```python
from build123d import *

# Parameters (mm, degrees)
SKETCH1_W           = 50
SKETCH1_H           = 50
BOSS_EXTRUDE1_DEPTH = 85
SKETCH2_R           = 5
BOSS_EXTRUDE2_DEPTH = 30
FILLET1_R           = 5
FILLET2_R           = 5
SKETCH3_W           = 70
SKETCH3_H           = 70
BOSS_EXTRUDE3_DEPTH = 10
FILLET3_R           = 5
SKETCH4_R           = 2.5
CUT_EXTRUDE1_DEPTH  = 10


with BuildPart() as part:
    # Sketch1 → Boss-Extrude1 (new body)
    with BuildSketch(Plane(origin=(0, 0, 0), x_dir=(1, 0, 0), z_dir=(0, 1, 0))):
        Rectangle(SKETCH1_W, SKETCH1_H)
    extrude(amount=BOSS_EXTRUDE1_DEPTH)

    # Sketch2 → Boss-Extrude2 (add)
    with BuildSketch(Plane.XZ):
        with Locations(Location((0, 0, 0), (0, 0, 90))):
            Circle(SKETCH2_R)
    extrude(amount=BOSS_EXTRUDE2_DEPTH)

    # Fillet1
    fillet1_edges = [part.edges().sort_by_distance(p)[0] for p in [
        (0, 85, 25),
        (0, 0, 25),
        (25, 42.5, 25),
        (-25, 42.5, 25),
    ]]
    fillet(fillet1_edges, radius=FILLET1_R)

    # Fillet2
    # the kernel refuses this fillet: 5 mm, written as the material it takes off along each edge
    with BuildSketch(Plane(origin=(-20, 80, 20), x_dir=(0, 1, 0), z_dir=(-1, 0, 0))) as fillet2_piece_1_section:
        Polygon((0, 0), (FILLET2_R, 0), (FILLET2_R, -FILLET2_R), (0, -FILLET2_R), align=None)
    fillet2_piece_1 = extrude(amount=FILLET2_R, mode=Mode.PRIVATE)
    fillet2_piece_1 = fillet2_piece_1 - Plane(origin=(-20, 80, 20), x_dir=(0, -0.7071067811865475, -0.7071067811865475), z_dir=(-1, 0, 0)) * Sphere(FILLET2_R, mode=Mode.PRIVATE)
    add(fillet2_piece_1, mode=Mode.SUBTRACT)
    with BuildSketch(Plane(origin=(20, 80, 20), x_dir=(1, 0, 0), z_dir=(0, 1, 0))) as fillet2_piece_2_section:
        Polygon((0, 0), (FILLET2_R, 0), (FILLET2_R, -FILLET2_R), (0, -FILLET2_R), align=None)
    fillet2_piece_2 = extrude(amount=FILLET2_R, mode=Mode.PRIVATE)
    fillet2_piece_2 = fillet2_piece_2 - Plane(origin=(20, 80, 20), x_dir=(-0.7071067811865475, 0, -0.7071067811865475), z_dir=(0, 1, 0)) * Sphere(FILLET2_R, mode=Mode.PRIVATE)
    add(fillet2_piece_2, mode=Mode.SUBTRACT)
    with BuildSketch(Plane(origin=(-20, 5, 20), x_dir=(0, -1, 0), z_dir=(-1, 0, 0))) as fillet2_piece_3_section:
        Polygon((0, 0), (FILLET2_R, 0), (FILLET2_R, FILLET2_R), (0, FILLET2_R), align=None)
    fillet2_piece_3 = extrude(amount=FILLET2_R, mode=Mode.PRIVATE)
    fillet2_piece_3 = fillet2_piece_3 - Plane(origin=(-20, 5, 20), x_dir=(0, 0.7071067811865475, -0.7071067811865475), z_dir=(-1, 0, 0)) * Sphere(FILLET2_R, mode=Mode.PRIVATE)
    add(fillet2_piece_3, mode=Mode.SUBTRACT)
    with BuildSketch(Plane(origin=(20, 5, 20), x_dir=(1, 0, 0), z_dir=(0, -1, 0))) as fillet2_piece_4_section:
        Polygon((0, 0), (FILLET2_R, 0), (FILLET2_R, FILLET2_R), (0, FILLET2_R), align=None)
    fillet2_piece_4 = extrude(amount=FILLET2_R, mode=Mode.PRIVATE)
    fillet2_piece_4 = fillet2_piece_4 - Plane(origin=(20, 5, 20), x_dir=(-0.7071067811865475, 0, -0.7071067811865475), z_dir=(0, -1, 0)) * Sphere(FILLET2_R, mode=Mode.PRIVATE)
    add(fillet2_piece_4, mode=Mode.SUBTRACT)
    with BuildSketch(Plane(origin=(-25, 85, 20), x_dir=(0, -1, 0), z_dir=(0, 0, -1)), Plane(origin=(25, 0, -37.5), x_dir=(-1, 0, 0), z_dir=(0, 0, 1))) as fillet2_piece_5:
        with BuildLine():
            CenterArc((FILLET2_R, -FILLET2_R), FILLET2_R, 90, 90)
            Line((0, -FILLET2_R), (0, 0))
            Line((0, 0), (FILLET2_R, 0))
        make_face()
    extrude(amount=57.5, mode=Mode.SUBTRACT)
    with BuildSketch(Plane(origin=(25, 85, -37.5), x_dir=(-1, 0, 0), z_dir=(0, 0, 1)), Plane(origin=(-25, 0, 20), x_dir=(0, 1, 0), z_dir=(0, 0, -1))) as fillet2_piece_6:
        with BuildLine():
            CenterArc((FILLET2_R, FILLET2_R), FILLET2_R, 180, 90)
            Line((0, FILLET2_R), (0, 0))
            Line((0, 0), (FILLET2_R, 0))
        make_face()
    extrude(amount=57.5, mode=Mode.SUBTRACT)

    # Sketch3 → Boss-Extrude3 (add)
    with BuildSketch(Plane.XZ):
        Rectangle(SKETCH3_W, SKETCH3_H)
    extrude(amount=-BOSS_EXTRUDE3_DEPTH)

    # Fillet3
    fillet3_edges = [part.edges().sort_by_distance(p)[0] for p in [
        (0, 85, -25),
        (-25, 45, -25),
        (25, 45, -25),
        (23.535533906, 83.535533906, -25),
        (-23.535533906, 83.535533906, -25),
    ]]
    fillet(fillet3_edges, radius=FILLET3_R)

    # Sketch4 → Cut-Extrude1 (cut)
    with BuildSketch(Plane.XZ):
        with Locations(Location((-30, 30, 0), (0, 0, 270))):
            Circle(SKETCH4_R)
        with Locations(Location((30, 30, 0), (0, 0, 270))):
            Circle(SKETCH4_R)
        with Locations(Location((30, -30, 0), (0, 0, 270))):
            Circle(SKETCH4_R)
        with Locations(Location((-30, -30, 0), (0, 0, 270))):
            Circle(SKETCH4_R)
    extrude(amount=-CUT_EXTRUDE1_DEPTH, mode=Mode.SUBTRACT)


solid = part.part
```
Here's how the part is built. I have some questions about the finished solid (model axes, mm). A direction names the side the tool comes from. Coordinates: 2 decimals unless noted, no trailing zeros. Loops run counter-clockwise (first coordinate to the right, second up) from the corner with the lowest first, then second, coordinate; pieces in that order, holes last. Notation, with made-up numbers: (77, 24.25) - (91, 24.25) arc R24 ccw to (91, 39.25) - close; hole circle Ø9 at (71.5, 35). An arc over 180 degrees is marked (long way). Return JSON: item names as keys, results as strings. Group by question number.
Item 1: If we section it at A-A on z = 30: Write out the boundary of the cut face in (x, y), and give its area (3 significant figures).
Item 2: If we section it at C-C on x = -30: Write out the boundary of the cut face in (y, z).
Item 3: Will these pins go through, and if not, where does the flat tip stop? P1, Ø8, axis at x = 30, z = 30, coming from the +Y side; P2, Ø2, axis at x = 20.5, y = 38, coming from the +Z side; P3, Ø10, axis at y = 65, z = 7.5, coming from the +X side.
Item 4: We'd pull the mould along Z, two halves only. Please class faces 1 (the face through (4.88, -14.79, -1.08)), 2 (the face through (-27.52, 4.93, -29.67)), 3 (the face through (23, 45, -24)): +Z half, -Z half, draft (parallel to the pull), parting line (faces both ways), or undercut.
Item 5: I need wall thicknesses on line 1 (X direction, y = 8, z = 30); line 2 (X direction, y = 33.5, z = -3). Which ranges of each line are inside material? Lowest first, please. Write a range as from..to.
Item 6: On a 3-axis mill with a long thin cutter (end or side, diameter ignored), from which of +Z, -Z, +X, -X, +Y, -Y can I reach the whole of each face in a straight line? I mean faces 4 (the face through (-24, 45, 23)), 5 (the face through (31.69, 4.93, 31.84)), 6 (the face through (23, 45, 24)), 7 (the face through (-23, 45, -24)), 8 (the face through (0, 45, -25)). Say none if no direction works.
Item 7: If we section it at B-B on y = 23.5: Write out the boundary of the cut face in (x, z), and give its area (3 significant figures).
Item 8: If we section it at D-D on z = 0: Write out the boundary of the cut face in (x, y), and give its area (3 significant figures).
Calculated:
{
 "1": {"outline": "(-35, 0) - (-32.5, 0) - (-32.5, 10) - (-35, 10) - close; (-27.5, 0) - (27.5, 0) - (27.5, 10) - (-27.5, 10) - close; (32.5, 0) - (35, 0) - (35, 10) - (32.5, 10) - close", "area": "600 mm^2"},
 "2": {"outline": "(0, -35) - (10, -35) - (10, -32.5) - (0, -32.5) - close; (0, -27.5) - (10, -27.5) - (10, 27.5) - (0, 27.5) - close; (0, 32.5) - (10, 32.5) - (10, 35) - (0, 35) - close"},
 "3": {"P1": "stops at y = 10", "P2": "stops at z = 25", "P3": "stops at x = 25"},
 "4": {"face 1": "parting line", "face 2": "undercut", "face 3": "-Z half"},
 "5": {"line 1": "x = -35..-32.5, -27.5..27.5, 32.5..35", "line 2": "x = -25..25"},
 "6": {"face 4": "+Z, -X, +Y", "face 5": "+Y, -Y", "face 6": "+Z, +X, +Y", "face 7": "-Z, -X, +Y", "face 8": "-Z, +X, -X, +Y"},
 "7": {"outline": "(-25, -20) arc R5 ccw to (-20, -25) - (20, -25) arc R5 ccw to (25, -20) - (25, 20) arc R5 ccw to (20, 25) - (-20, 25) arc R5 ccw to (-25, 20) - close", "area": "2,480 mm^2"},
 "8": {"outline": "(-35, 0) - (-5, 0) - (-5, -30) - (5, -30) - (5, 0) - (35, 0) - (35, 10) - (25, 10) - (25, 80) arc R5 ccw to (20, 85) - (-20, 85) arc R5 ccw to (-25, 80) - (-25, 10) - (-35, 10) - close", "area": "4,740 mm^2"}
}
